Design review of the part built by this model. Coordinates are the model's own, in mm. A direction names the side the tool comes from. Coordinates: 2 decimals unless noted, no trailing zeros. Loops run counter-clockwise (first coordinate to the right, second up) from the corner with the lowest first, then second, coordinate; pieces in that order, holes last. Notation, with made-up numbers: (69, 87.25) -> (125, 87.25) arc R27 ccw to (125, 115.25) -> close; hole circle Ø3 at (-31, 16). An arc over 180 degrees is marked (long way). Use a Markdown table: item, result. Add a question column.
Q1. Take a section at C-C on y = 5.5. Write out the cut boundary in (x, z).
Q2. For probe 1 along Y at (x, z) = (0, 14.5); probe 2 along Y at (x, z) = (-0.5, 13.5); probe 3 along Z at (x, y) = (2.5, 6), list the stretches that pass through material, from the lowest coordinate up.
Q3. Take a section at B-B on z = 14.5. Write out the cut boundary in (x, y).
Q4. Take a section at A-A on z = 23.25. Write out the cut boundary in (x, y), plus the area to 3 significant figures.
Q5. For faces 1 (the face through (0, 2, 25)), 2 (the face through (0.07, 9.582, 15.581)), list the 3-axis set-ups (+Z, -Z, +X, -X, +Y, -Y) from which the entire face can be reached by the end or side of a thin tool; tool diameter is ignored.
Q6. Clearance check with flat-ended pins moving along their axes: pin 1 Ø5 at (x, y) = (2, 8) entering from -Z; pin 2 Ø12 at (y, z) = (-10.21, 12.5) entering from -X; pin 3 Ø3.5 at (x, y) = (0, 16.41) entering from +Z. State where each tip first meets the part, or that it passes through.
Q7. Take a section at D-D on z = 7.75. Write out the cut boundary in (x, y).
Q8. Draft analysis for pull direction X (two halves, no side actions). For faces 3 (the face through (2.41, -13.25, 9.55)), 4 (the face through (-1.129, 18.184, 17.699)), 5 (the face through (-2.46, -13.07, 9.55)), state which applies: pulls with the +X half, pulls with the -X half, needs draft (parallel to the pull), parting line crosses it, or undercut.
from build123d import *

# Parameters (mm, degrees)
F0_W     = 10
F0_H     = 20
F1_DEPTH = 25
F3_DEPTH = 10.001
F4_R     = 3.75
F5_DEPTH = 12.5
F7_D     = 4.2
F7_DEPTH = 14.4
F7_TIP   = 1.2618073


with BuildPart() as f1:
    # F0 (on Top) → F1 (new body)
    with BuildSketch(Plane.XY):
        with BuildLine():
            Line((1.4488887394, -16.8391867264), (5, -3.5862590786))
            Line((5, -3.5862590786), (-5, -3.5862590786))
            Line((-5, -3.5862590786), (-1.4488887394, -16.8391867264))
            ThreePointArc((-1.4488887394, -16.8391867264), (0, -17.9509581587), (1.4488887394, -16.8391867264))
        make_face()
        with Locations((0, 6.4137409214)):
            Rectangle(F0_W, F0_H)
        with BuildLine():
            Line((-5, 16.4137409214), (5, 16.4137409214))
            ThreePointArc((5, 16.4137409214), (0, 21.4137409214), (-5, 16.4137409214))
        make_face()
    extrude(amount=F1_DEPTH)

    # F2 (on face) → F3 (cut, through all)
    with BuildSketch(Plane.YZ.offset(5)):
        Polygon((12.6637409214, 12.5), (6.4137409214, 18.75), (-2.5862590786, 12.5), (6.4137409214, 6.25), align=None)
    extrude(amount=-F3_DEPTH, mode=Mode.SUBTRACT)

    # F4 (on Right) → F5 (cut, symmetric)
    with BuildSketch(Plane.YZ):
        with Locations((-10.2127229025, 12.5)):
            Circle(F4_R)
    extrude(amount=F5_DEPTH, both=True, mode=Mode.SUBTRACT)

    # F7
    with Locations(Plane.XY.offset(25)):
        with Locations((0, 16.4137409214)):
            Hole(F7_D / 2, depth=F7_DEPTH)
            with Locations((0, 0, -(F7_DEPTH + F7_TIP / 2))):  # 118° drill point
                Cone(0, F7_D / 2, F7_TIP, mode=Mode.SUBTRACT)


solid = f1.part
Answer list:
| question | item | result |
|---|---|---|
| 1 | outline | (-5, 0) -> (5, 0) -> (5, 6.88) -> (-5, 6.88) -> close; (-5, 18.12) -> (5, 18.12) -> (5, 25) -> (-5, 25) -> close |
| 2 | probe 1 | -17.95 to -13.38, -7.04 to 0.29, 10.66 to 14.31, 18.51 to 21.41 |
| 2 | probe 2 | -17.87 to -13.83, -6.6 to -1.15, 11.66 to 14.37, 18.45 to 21.39 |
| 2 | probe 3 | 0 to 6.54, 18.46 to 25 |
| 3 | outline | (-5, -3.59) -> (-4.07, -7.04) -> (4.07, -7.04) -> (5, -3.59) -> (5, 0.29) -> (-5, 0.29) -> close; (-5, 10.66) -> (5, 10.66) -> (5, 16.41) arc R5 ccw to (-5, 16.41) -> close; (-2.37, -13.38) -> (-1.45, -16.84) arc R1.5 ccw to (1.45, -16.84) -> (2.37, -13.38) -> close; hole circle Ø4.2 at (0, 16.41) |
| 4 | outline | (-5, -3.59) -> (-1.45, -16.84) arc R1.5 ccw to (1.45, -16.84) -> (5, -3.59) -> (5, 16.41) arc R5 ccw to (-5, 16.41) -> close; hole circle Ø4.2 at (0, 16.41) |
| 4 | area | 313 mm² |
| 5 | face 1 | +Z, +X, -X, +Y, -Y |
| 5 | face 2 | +X, -X |
| 6 | pin 1 | z = 0 |
| 6 | pin 2 | x = -4.83 |
| 6 | pin 3 | z = 10.39 |
| 7 | outline | (-5, -3.59) -> (-1.45, -16.84) arc R1.5 ccw to (1.45, -16.84) -> (5, -3.59) -> (5, 4.25) -> (-5, 4.25) -> close; (-5, 7.91) -> (5, 7.91) -> (5, 16.41) arc R5 ccw to (-5, 16.41) -> close |
| 8 | face 3 | pulls with the +X half |
| 8 | face 4 | undercut |
| 8 | face 5 | pulls with the -X half |
